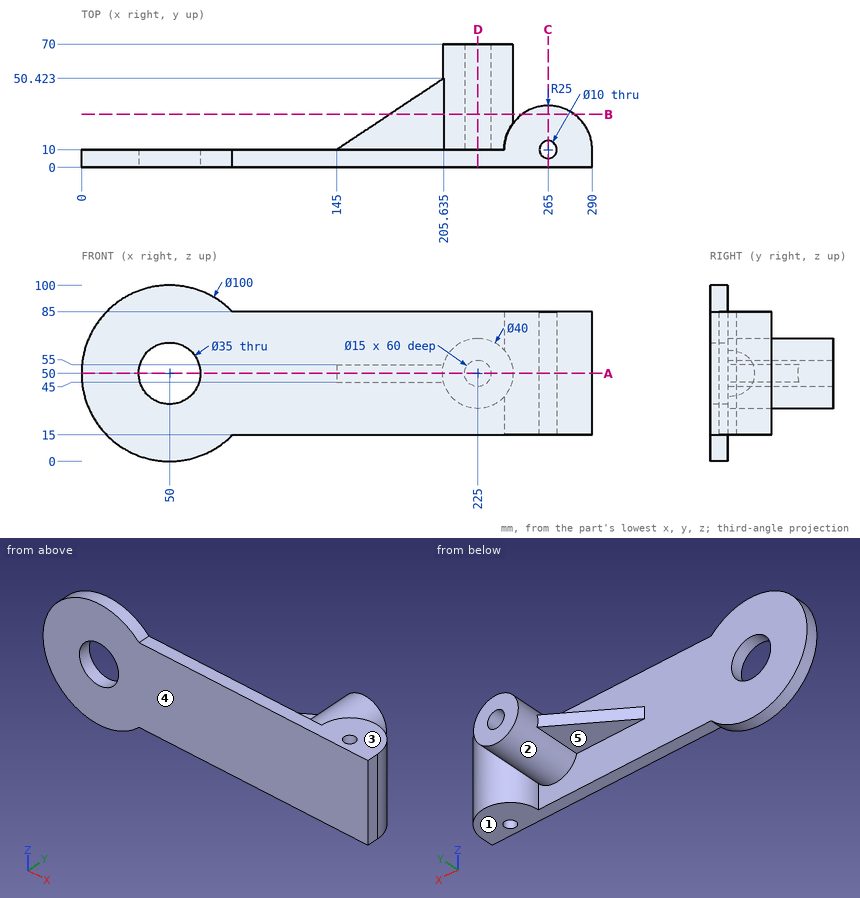
Job drawing, mm, ordinate dimensions from the low corner. One solid piece. A direction names the side the tool comes from. Round coordinates to 2 decimals unless told otherwise and drop trailing zeros. Write each loop counter-clockwise with the first axis right and the second up, starting at its lowest first coordinate (ties: lowest second). Pieces come first, ordered by that corner, then holes. Notation, with made-up numbers: (68.25, 17) -> (78.25, 17) arc R30 ccw to (78.25, 53) -> close; hole circle Ø7 at (13, 48). An arc over 180 degrees is marked (long way). Answer as a JSON object with one key per item and string values.
(1) Pin check, flat tips, straight feed: P1, Ø3, axis at x = 98, z = 18.5, coming from the +Y side; P2, Ø12, axis at x = 178, y = 28, coming from the -Z side; P3, Ø17.5, axis at x = 221.5, y = 15.5, coming from the +Z side. Stop position of each tip, or through.
Reported:
{"P1": "stops at y = 10", "P2": "stops at z = 45", "P3": "stops at z = 85"}
(2) Band-saw the part on D-D, the plane x = 225. List the corners of the cut face in (y, z), then the cut area to 3 significant figures.
Reported:
{"outline": "(0, 15) -> (10, 15) -> (10, 30) -> (70, 30) -> (70, 42.5) -> (10, 42.5) -> (10, 57.5) -> (70, 57.5) -> (70, 70) -> (10, 70) -> (10, 85) -> (0, 85) -> close", "area": "2,200 mm^2"}
(3) Probe probe 1 along Z at (x, y) = (225, 42); probe 2 along X at (y, z) = (32, 50) (1 decimal); probe 3 along Z at (x, y) = (203.5, 32). List the from-to ranges inside material, lowest first. Write a range as [from, to].
Reported:
{"probe 1": "z = [30, 42.5], [57.5, 70]", "probe 2": "x = [178, 217.5], [232.5, 245], [253.1, 276.9]", "probe 3": "z = [45, 55]"}
(4) Band-saw the part on A-A, the plane z = 50. List the corners of the cut face in (x, y).
Reported:
{"outline": "(0, 0) -> (32.5, 0) -> (32.5, 10) -> (0, 10) -> close; (67.5, 0) -> (290, 0) -> (290, 10) arc R25 ccw to (245, 25) -> (245, 70) -> (232.5, 70) -> (232.5, 10) -> (217.5, 10) -> (217.5, 70) -> (205, 70) -> (205, 50) -> (145, 10) -> (67.5, 10) -> close; hole circle Ø10 at (265, 10)"}
(5) Two-plate mould, pull along X, no slides. Class the marked faces 1 and 2: +X half, -X half, draft (parallel to the pull), parting line (faces both ways), or undercut.
Reported:
{"face 1": "draft", "face 2": "undercut"}
(6) Which spindle directions (+Z, -Z, +X, -X, +Y, -Y) get a long thin tool onto all of the face, cutting with end or side? Do the marked faces 3, 4 and 5. Say none if no direction does.
Reported:
{"face 3": "+Z, +X, +Y, -Y", "face 4": "+Z, -Z, +X, -X, -Y", "face 5": "-Z, -X, +Y"}
(7) Band-saw the part on C-C, the plane x = 265. List the corners of the cut face in (y, z), then the cut area to 3 significant figures.
Reported:
{"outline": "(0, 15) -> (5, 15) -> (5, 85) -> (0, 85) -> close; (15, 15) -> (35, 15) -> (35, 85) -> (15, 85) -> close", "area": "1,750 mm^2"}
(8) Band-saw the part on B-B, the plane y = 30. List the corners of the cut face in (x, z) (1 decimal).
Reported:
{"outline": "(175, 45) -> (205.6, 45) arc R20 ccw (long way) to (205.6, 55) -> (175, 55) -> close; (250, 15) -> (280, 15) -> (280, 85) -> (250, 85) -> close; hole circle Ø15 at (225, 50)"}
